Model file for the job. Use its own axes, mm. A direction names the side the tool comes from. Round coordinates to 2 decimals unless told otherwise and drop trailing zeros. Loops run counter-clockwise (first coordinate to the right, second up) from the corner with the lowest first, then second, coordinate; pieces in that order, holes last. Notation, with made-up numbers: M -29.5,-8 L 6.5,-8 A29 cw 6.5,18 Z; hole C -30,-17 d5. An arc over 180 degrees is marked long. Use a Markdown table: item, result. Add a question column.
Q1. Cut at A-A (z = 21.5). Give the cut face in (x, y), plus the area to 3 significant figures.
Q2. Pin check, flat tips, straight feed: pin 1 (19.5 mm diameter, centred on x = -9.5, z = 3.5, fed in from +Y); pin 2 (1.5 mm diameter, centred on x = -6.5, y = 6.5, fed in from -Z); pin 3 (4.5 mm diameter, centred on x = 1.5, y = 2.5, fed in from +Z); pin 4 (2 mm diameter, centred on x = 15.5, z = -7.5, fed in from +Y). Stop position of each tip, or through.
Q3. Mould opens along X. For faces 1 (the face through (-21.99, 1.48, -2.23)), 2 (the face through (12.927, 6.768, -0.358)), 3 (the face through (0, 5, 12.5)) say: +X half, -X half, draft (parallel to the pull), parting line (faces both ways), or undercut.
Q4. Cut at C-C (x = 8). Give the cut face in (y, z), plus the area to 3 significant figures.
Q5. Tool access for faces 4 (the face through (10, 5.5, 0)), 5 (the face through (-10, 7, 0)), 6 (the face through (0, 3, 16.5)), 7 (the face through (0, 1, -12)): list every direction of +Z, -Z, +X, -X, +Y, -Y with a clear straight run to the whole face (end or side of a thin tool).
Q6. Cut at D-D (x = 0). Give the cut face in (y, z), plus the area to 3 significant figures.
Q7. Probe line 1 (X direction, y = 7.1, z = 21.5); line 2 (X direction, y = 7.25, z = 0); line 3 (Y direction, x = -16, z = 4.5). List the from-to ranges inside material, lowest first. Write a range as from..to.
Q8. Cut at B-B (z = 0). Give the cut face in (x, y).
from build123d import *

# Parameters (mm, degrees)
BOSS_EXTRU_1_DEPTH      = 3
ESQUISSE2_R             = 3.75
BOSS_EXTRU_2_DEPTH      = 5
ESQUISSE4_W             = 30
ESQUISSE4_H             = 4
BOSS_EXTRU_3_DEPTH      = 5
ESQUISSE5_W             = 30
ESQUISSE5_H             = 2.5
BOSS_EXTRU_4_DEPTH      = 10
ESQUISSE6_R             = 2.05
ENL_V_MAT_EXTRU_3_DEPTH = 10
ESQUISSE7_R             = 2.75
ENL_V_MAT_EXTRU_4_DEPTH = 2.5
ESQUISSE8_R             = 3.75
BOSS_EXTRU_5_DEPTH      = 4
CONG_1_R                = 1.5


with BuildPart() as part:
    # Esquisse1 → Boss.-Extru.1 (new body)
    with BuildSketch(Plane(origin=(0, 0, 0), x_dir=(1, 0, 0), z_dir=(0, 1, 0))):
        with BuildLine():
            Line((-10.2, 12), (10.2, 12))
            ThreePointArc((10.2, 12), (21.946875755, 2.451715724), (15, -10.998181668))
            Line((15, -10.998181668), (15, -16.5))
            Line((15, -16.5), (-15, -16.5))
            Line((-15, -16.5), (-15, -10.998181668))
            ThreePointArc((-15, -10.998181668), (-21.946875755, 2.451715724), (-10.2, 12))
        make_face()
    extrude(amount=BOSS_EXTRU_1_DEPTH)

    # Esquisse2 → Boss.-Extru.2 (add)
    with BuildSketch(Plane(origin=(0, 3, 0), x_dir=(1, 0, 0), z_dir=(0, 1, 0))):
        with Locations(Location((10.2, 0, 0), (0, 0, 270))):
            Circle(ESQUISSE2_R)
    extrude(amount=BOSS_EXTRU_2_DEPTH)

    # Esquisse4 → Boss.-Extru.3 (add)
    with BuildSketch(Plane(origin=(0, 3, 0), x_dir=(1, 0, 0), z_dir=(0, 1, 0))):
        with Locations((0, -14.5)):
            Rectangle(ESQUISSE4_W, ESQUISSE4_H)
    extrude(amount=BOSS_EXTRU_3_DEPTH)

    # Esquisse5 → Boss.-Extru.4 (add)
    with BuildSketch(Plane.XY.offset(16.5)):
        with Locations((0, 6.75)):
            Rectangle(ESQUISSE5_W, ESQUISSE5_H)
    extrude(amount=BOSS_EXTRU_4_DEPTH)

    # Esquisse6 → Enlèv. mat.-Extru.3 (cut)
    with BuildSketch(Plane(origin=(0, 8, 0), x_dir=(1, 0, 0), z_dir=(0, 1, 0))):
        with Locations(Location((8, -21.5, 0), (0, 0, 270))):
            Circle(ESQUISSE6_R)
        with Locations(Location((-8, -21.5, 0), (0, 0, 270))):
            Circle(ESQUISSE6_R)
    extrude(amount=-ENL_V_MAT_EXTRU_3_DEPTH, mode=Mode.SUBTRACT)

    # Esquisse7 → Enlèv. mat.-Extru.4 (cut)
    with BuildSketch(Plane(origin=(0, 8, 0), x_dir=(1, 0, 0), z_dir=(0, 1, 0))):
        with Locations(Location((10.2, 0, 0), (0, 0, 270))):
            Circle(ESQUISSE7_R)
    extrude(amount=-ENL_V_MAT_EXTRU_4_DEPTH, mode=Mode.SUBTRACT)

    # Esquisse8 → Boss.-Extru.5 (add)
    with BuildSketch(Plane(origin=(0, 3, 0), x_dir=(1, 0, 0), z_dir=(0, 1, 0))):
        with Locations(Location((-10.2, 0, 0), (0, 0, 270))):
            Circle(ESQUISSE8_R)
    extrude(amount=BOSS_EXTRU_5_DEPTH)

    # Congé1
    cong_1_edges = [part.edges().sort_by_distance(p)[0] for p in [
        (0, 0, 16.5),
    ]]
    fillet(cong_1_edges, radius=CONG_1_R)


solid = part.part
Checked values:
| question | item | result |
|---|---|---|
| 1 | outline | M -15,5.5 L -10.05,5.5 L -10.05,8 L -15,8 Z; M -5.95,5.5 L 5.95,5.5 L 5.95,8 L -5.95,8 Z; M 10.05,5.5 L 15,5.5 L 15,8 L 10.05,8 Z |
| 1 | area | 54.5 mm^2 |
| 2 | pin 1 | stops at y = 8 |
| 2 | pin 2 | stops at z = -2.32 |
| 2 | pin 3 | stops at z = 16.5 |
| 2 | pin 4 | stops at y = 3 |
| 3 | face 1 | -X half |
| 3 | face 2 | undercut |
| 3 | face 3 | draft |
| 4 | outline | M 0,-12 L 3,-12 L 3,-3.04 L 8,-3.04 L 8,-1.65 L 5.5,-1.65 L 5.5,1.65 L 8,1.65 L 8,3.04 L 3,3.04 L 3,12.5 L 8,12.5 L 8,19.45 L 5.5,19.45 L 5.5,16.5 L 1.5,16.5 A1.5 ccw 0,15 Z; M 5.5,23.55 L 8,23.55 L 8,26.5 L 5.5,26.5 Z |
| 4 | area | 142 mm^2 |
| 5 | face 4 | +Y |
| 5 | face 5 | -Z, -X, +Y |
| 5 | face 6 | +Z, +X, -X, -Y |
| 5 | face 7 | -Z, +X, -X, +Y, -Y |
| 6 | outline | M 0,-12 L 3,-12 L 3,12.5 L 8,12.5 L 8,26.5 L 5.5,26.5 L 5.5,16.5 L 1.5,16.5 A1.5 ccw 0,15 Z |
| 6 | area | 130 mm^2 |
| 7 | line 1 | x = -15..-10.05, -5.95..5.95, 10.05..15 |
| 7 | line 2 | x = 6.45..7.45, 12.95..13.95 |
| 7 | line 3 | y = 0..3 |
| 8 | outline | M -22.2,0 L 22.2,0 L 22.2,3 L 13.95,3 L 13.95,8 L 12.95,8 L 12.95,5.5 L 7.45,5.5 L 7.45,8 L 6.45,8 L 6.45,3 L -6.45,3 L -6.45,7 L -13.95,7 L -13.95,3 L -22.2,3 Z |
